from build123d import *

# Parameters (mm, degrees)
SKETCH1_W           = 20
SKETCH1_H           = 20
BOSS_EXTRUDE1_DEPTH = 10
SKETCH2_R           = 3
CUT_EXTRUDE1_DEPTH  = 11
SKETCH3_R           = 1.6
CUT_EXTRUDE2_DEPTH  = 11
CHAMFER1_SIZE       = 1
CHAMFER2_SIZE       = 1
SKETCH5_R           = 3.025
SKETCH5_R_2         = 1
SKETCH5_R_3         = 1.5
CUT_EXTRUDE3_DEPTH  = 21
SKETCH2_3_R         = 1.5
CUT_EXTRUDE4_DEPTH  = 4


with BuildPart() as part:
    # Sketch1 → Boss-Extrude1 (new body)
    with BuildSketch(Plane(origin=(0, 0, 0), x_dir=(1, 0, 0), z_dir=(0, 1, 0))):
        Rectangle(SKETCH1_W, SKETCH1_H)
    extrude(amount=-BOSS_EXTRUDE1_DEPTH)

    # Sketch2 → Cut-Extrude1 (cut, through all)
    with BuildSketch(Plane(origin=(0, 0, 0), x_dir=(1, 0, 0), z_dir=(0, 1, 0))):
        with Locations((0, 4)):
            Circle(SKETCH2_R)
    extrude(amount=-CUT_EXTRUDE1_DEPTH, mode=Mode.SUBTRACT)

    # Sketch3 → Cut-Extrude2 (cut, through all)
    with BuildSketch(Plane(origin=(0, 0, 0), x_dir=(1, 0, 0), z_dir=(0, 1, 0))):
        with Locations((7, 5.5)):
            Circle(SKETCH3_R)
    cut_extrude2 = extrude(amount=-CUT_EXTRUDE2_DEPTH, mode=Mode.SUBTRACT)

    # Mirror1: Cut-Extrude2 across plane
    add(cut_extrude2.mirror(Plane(origin=(0, 0, 0), x_dir=(0, 0, 1), z_dir=(1, 0, 0))), mode=Mode.SUBTRACT)

    # Chamfer1
    chamfer1_edges = [part.edges().sort_by_distance(p)[0] for p in [
        (5.4, -10, -5.5),
    ]]
    chamfer(chamfer1_edges, length=CHAMFER1_SIZE)

    # Chamfer2
    chamfer2_edges = [part.edges().sort_by_distance(p)[0] for p in [
        (-5.4, -10, -5.5),
    ]]
    chamfer(chamfer2_edges, length=CHAMFER2_SIZE)

    # Sketch5 → Cut-Extrude3 (cut, through all)
    with BuildSketch(Plane(origin=(10, 0, 0), x_dir=(0, 0, -1), z_dir=(1, 0, 0))):
        with Locations((-5.5, -5)):
            Circle(SKETCH5_R)
        with Locations((1.5, -8)):
            Circle(SKETCH5_R_2)
        with Locations((1.5, -4.5)):
            Circle(SKETCH5_R_3)
    extrude(amount=-CUT_EXTRUDE3_DEPTH, mode=Mode.SUBTRACT)

    # Sketch2<3> → Cut-Extrude4 (cut)
    with BuildSketch(Plane(origin=(0, 0, 0), x_dir=(1, 0, 0), z_dir=(0, 1, 0))):
        with Locations((0, -5.5)):
            Circle(SKETCH2_3_R)
    extrude(amount=-CUT_EXTRUDE4_DEPTH, mode=Mode.SUBTRACT)


solid = part.part
The model under review builds one solid part; all positions refer to its coordinate system, in mm. A direction names the side the tool comes from. Round coordinates to 2 decimals unless told otherwise and drop trailing zeros. Loops run counter-clockwise (first coordinate to the right, second up) from the corner with the lowest first, then second, coordinate; pieces in that order, holes last. Notation, with made-up numbers: M 31.25,83 L 38.25,83 A20 cw 38.25,90 Z; hole C 34,26.25 d3. An arc over 180 degrees is marked long. Answer as a JSON object with one key per item and string values.
Item 1: Clearance check with a flat-ended pin moving along its axis: P1, Ø4, axis at x = -7, z = -5.5, coming from the -Y side. State where the tip first meets the part, or that it passes through.
Check sheet entries:
{"P1": "y = -9.4"}
Item 2: The part is to be moulded in two halves that separate along X. For faces 1 (the face through (-10, -4.93, 0.14)), 2 (the face through (5.73, -4.44, -4.53)), 3 (the face through (0.14, -7.953, 6.156)), say which applies: +X half, -X half, draft (parallel to the pull), parting line (faces both ways), or undercut.
Check sheet entries:
{"face 1": "-X half", "face 2": "undercut", "face 3": "draft"}
Item 3: We need section C-C, the plane y = -4.5. State the section outline as (x, z) points.
Check sheet entries:
{"outline": "M -10,-10 L 10,-10 L 10,-3 L 2.83,-3 A3 cw long -2.83,-3 L -10,-3 Z; M -10,0 L 10,0 L 10,2.52 L -10,2.52 Z; M -10,8.48 L 10,8.48 L 10,10 L -10,10 Z; hole C -7,-5.5 d3.2; hole C 7,-5.5 d3.2"}
Item 4: Tool access review of faces 4 (the face through (1.43, -1.17, 5.05)), 5 (the face through (-5.73, -4.44, -4.53)): name each direction out of +Z, -Z, +X, -X, +Y, -Y from which nothing blocks a thin tool from reaching the whole face with its end or side.
Check sheet entries:
{"face 4": "+Y", "face 5": "+Y, -Y"}
Item 5: We need section D-D, the plane y = -1.5. State the section outline as (x, z) points, and give its area (3 significant figures).
Check sheet entries:
{"outline": "M -10,-10 L 10,-10 L 10,10 L -10,10 Z; hole C -7,-5.5 d3.2; hole C 0,-4 d6; hole C 0,5.5 d3; hole C 7,-5.5 d3.2", "area": "349 mm2"}
Item 6: We need section B-B, the plane z = 5.5. State the section outline as (x, y) points (3 decimals).
Check sheet entries:
{"outline": "M -10,-10 L 10,-10 L 10,-8.025 L -10,-8.025 Z; M -10,-1.975 L -1.5,-1.975 L -1.5,0 L -10,0 Z; M 1.5,-1.975 L 10,-1.975 L 10,0 L 1.5,0 Z"}
Item 7: For line 1 along Z through (x, y) = (0, -1.75); line 2 along Y through (x, z) = (3.5, -1.5); line 3 along Y through (x, z) = (-3.25, 5.5) (3 decimals), list the stretches that pass through material, from the lowest coordinate up.
Check sheet entries:
{"line 1": "-10 to -7, -1 to 4, 7 to 10", "line 2": "-10 to -9, -7 to -6, -3 to 0", "line 3": "-10 to -8.025, -1.975 to 0"}
Item 8: We need section A-A, the plane x = 7. State the section outline as (y, z) points (3 decimals), and give its area (3 significant figures).
Check sheet entries:
{"outline": "M -10,-10 L 0,-10 L 0,-7.1 L -9,-7.1 L -10,-8.1 Z; M -10,-2.9 L -9,-3.9 L 0,-3.9 L 0,10 L -10,10 Z; hole C -8,-1.5 d2; hole C -5,5.5 d6.05; hole C -4.5,-1.5 d3", "area": "128 mm2"}
